CAD build for the part. Positions are in the model's coordinates, mm. A direction names the side the tool comes from. Round coordinates to 2 decimals unless told otherwise and drop trailing zeros. Loops run counter-clockwise (first coordinate to the right, second up) from the corner with the lowest first, then second, coordinate; pieces in that order, holes last.
```python
from build123d import *

# Parameters (mm, degrees)
SKETCH1_W                       = 69.85
SKETCH1_H                       = 25.4
BASE_FLANGE1_DEPTH              = 4.55422
F_7_32_0_21875_DIAMETER_HOLE1_D = 5.55625
BREAK_CORNER1_DEPTH             = 4.55422
SKETCH4_W                       = 34.925
SKETCH4_H                       = 3.175
TAB1_DEPTH                      = 4.55422
FILLET1_R                       = 9.525
CUT_EXTRUDE1_REACH              = 40.633
SKETCH7_R                       = 9.525
CUT_EXTRUDE3_DEPTH              = 2.38125
F_9_32_0_28125_DIAMETER_HOLE1_D = 7.14375
FILLET3_R                       = 12.7
CUT_EXTRUDE4_START              = -2.17297
CUT_EXTRUDE4_DEPTH              = 2.17297


# Read off the part's stored shape, not the designer's step: Break-Corner1
# Sheet-metal steps are written as plain solids
with BuildPart() as part:
    # Sketch1 → Base-Flange1 (new body)
    with BuildSketch(Plane.XY):
        Rectangle(SKETCH1_W, SKETCH1_H)
    extrude(amount=BASE_FLANGE1_DEPTH)

    # 7/32 (0.21875) Diameter Hole1 (through all)
    with Locations(Plane.XY.offset(4.55422)):
        with Locations((-28.575, 6.35), (-28.575, -6.35), (28.575, 6.35), (28.575, -6.35)):
            Hole(F_7_32_0_21875_DIAMETER_HOLE1_D / 2)

    # Break-Corner1 outline → Break-Corner1 (cut)
    with BuildSketch(Plane.XY):
        with BuildLine():
            Line((34.925, -12.7), (34.925, -9.525))
            ThreePointArc((34.925, -9.525), (33.99506403, -11.77006403), (31.75, -12.7))
            Line((31.75, -12.7), (34.925, -12.7))
        make_face()
        with BuildLine():
            ThreePointArc((31.75, 12.7), (33.99506403, 11.77006403), (34.925, 9.525))
            Line((34.925, 9.525), (34.925, 12.7))
            Line((34.925, 12.7), (31.75, 12.7))
        make_face()
        with BuildLine():
            Line((-34.925, -12.7), (-31.75, -12.7))
            ThreePointArc((-31.75, -12.7), (-33.99506403, -11.77006403), (-34.925, -9.525))
            Line((-34.925, -9.525), (-34.925, -12.7))
        make_face()
        with BuildLine():
            ThreePointArc((-34.925, 9.525), (-33.99506403, 11.77006403), (-31.75, 12.7))
            Line((-31.75, 12.7), (-34.925, 12.7))
            Line((-34.925, 12.7), (-34.925, 9.525))
        make_face()
    extrude(amount=BREAK_CORNER1_DEPTH, mode=Mode.SUBTRACT)

    # Sketch4 → Tab1 (add)
    with BuildSketch(Plane(origin=(0, 0, 0), x_dir=(-1, 0, 0), z_dir=(0, 0, -1))):
        with Locations((0, -14.2875)):
            Rectangle(SKETCH4_W, SKETCH4_H)
    extrude(amount=-TAB1_DEPTH)

    # Fillet1
    # the kernel refuses this fillet: 9.525 mm, written as the material it adds along each edge
    with BuildSketch(Plane(origin=(-17.4625, -12.7, 0), x_dir=(-1, 0, 0), z_dir=(0, 0, 1))) as fillet1_piece_1:
        with BuildLine():
            CenterArc((7.099515829, 9.525), FILLET1_R, 221.810314896, 48.189685104)
            Line((0, 3.175), (-0.141990317, 3.048))
            ThreePointArc((-0.141990317, 3.048), (-0.1905, 1.5875), (-0.1905, 0))
            Line((-0.1905, 0), (0, -0.1905))
            Line((0, -0.1905), (7.099515829, -0.1905))
            Line((7.099515829, -0.1905), (7.099515829, 0))
        make_face()
    extrude(amount=4.55422)
    with BuildSketch(Plane(origin=(17.4625, -12.7, 0), x_dir=(1, 0, 0), z_dir=(0, 0, 1))) as fillet1_piece_2:
        with BuildLine():
            CenterArc((7.099515829, -9.525), FILLET1_R, 90, 48.189685104)
            Line((0, -3.175), (-0.141990317, -3.048))
            ThreePointArc((-0.141990317, -3.048), (-0.1905, -1.5875), (-0.1905, 0))
            Line((-0.1905, 0), (0, 0.1905))
            Line((0, 0.1905), (7.099515829, 0.1905))
            Line((7.099515829, 0.1905), (7.099515829, 0))
        make_face()
    extrude(amount=4.55422)

    # Sketch5 → Cut-Extrude1 (cut, up to next)
    with BuildSketch(Plane(origin=(0, 0, 0), x_dir=(-1, 0, 0), z_dir=(0, 0, -1)), mode=Mode.PRIVATE) as cut_extrude1_sk1:
        with BuildLine():
            Line((-8.064231886, 9.525), (8.064231886, 9.525))
            ThreePointArc((8.064231886, 9.525), (9.864287689, 9.69663568), (11.599471303, 10.205357143))
            ThreePointArc((11.599471303, 10.205357143), (17.961811219, 12.070669174), (24.562015829, 12.7))
            Line((24.562015829, 12.7), (-24.562015829, 12.7))
            ThreePointArc((-24.562015829, 12.7), (-17.961811219, 12.070669174), (-11.599471303, 10.205357143))
            ThreePointArc((-11.599471303, 10.205357143), (-9.864287689, 9.69663568), (-8.064231886, 9.525))
        make_face()
    cut_extrude1_tool1 = extrude(cut_extrude1_sk1.sketch, amount=-CUT_EXTRUDE1_REACH, mode=Mode.PRIVATE) & part.part
    add(cut_extrude1_tool1.solids().sort_by_distance((0, 11.328032, 0))[0], mode=Mode.SUBTRACT)

    # Sketch7 → Cut-Extrude3 (cut)
    with BuildSketch(Plane(origin=(0, 0, 0), x_dir=(-1, 0, 0), z_dir=(0, 0, -1))):
        with Locations((0, -3.175)):
            Circle(SKETCH7_R)
    extrude(amount=-CUT_EXTRUDE3_DEPTH, mode=Mode.SUBTRACT)

    # 9/32 (0.28125) Diameter Hole1 (through all)
    with Locations(Plane(origin=(0, 0, 2.38125), x_dir=(-1, 0, 0), z_dir=(0, 0, -1))):
        with Locations((0, -3.175)):
            Hole(F_9_32_0_28125_DIAMETER_HOLE1_D / 2)

    # Fillet3
    fillet3_edges = [part.edges().sort_by_distance(p)[0] for p in [
        (17.4625, -15.875, 2.27711),
        (-17.4625, -15.875, 2.27711),
    ]]
    fillet(fillet3_edges, radius=FILLET3_R)

    # Sketch10 → Cut-Extrude4 (cut)
    with BuildSketch(Plane.XY.offset(4.55422).offset(CUT_EXTRUDE4_START)):
        with BuildLine():
            Line((3.571875, -2.38125), (3.571875, -5.55625))
            ThreePointArc((3.571875, -5.55625), (0, -9.128125), (-3.571875, -5.55625))
            Line((-3.571875, -5.55625), (-3.571875, -2.38125))
            ThreePointArc((-3.571875, -2.38125), (0, 1.190625), (3.571875, -2.38125))
        make_face()
    extrude(amount=CUT_EXTRUDE4_DEPTH, mode=Mode.SUBTRACT)


solid = part.part
```
Item 1: Flat gauge pins, fed straight in: P1, Ø1.4, axis at x = -1, z = 1.5, coming from the +Y side (3 decimals); P2, Ø5.5, axis at x = 3, y = -1, coming from the -Z side; P3, Ø2, axis at x = 26, z = 0.5, coming from the -Y side; P4, Ø4.5, axis at x = 28.575, y = -6.35, coming from the +Z side. Where does each tip first touch, or does it go through?
Answers follow:
P1: stops at y = 9.525
P2: stops at z = 2.38
P3: stops at y = -12.7
P4: passes through
Item 2: 3-axis set-ups, long thin cutter, end or side, ignore diameter. For faces 1 (the cylindrical face through (2.065, -12.473, 1.174)), 2 (the flat face through (28, -12.7, 2)), 3 (the flat face through (-3.572, -4, 3)), 4 (the flat face through (-28, -12.7, 2)): which of +Z, -Z, +X, -X, +Y, -Y reach the whole face in a straight line?
Answers follow:
face 1: -Z
face 2: +Z, -Z, +X, -Y
face 3: +Z, -Z
face 4: +Z, -Z, -X, -Y
Item 3: Cut at D-D, the plane y = -0.5. Give the cut face in (x, z) (3 decimals), plus the area to 3 significant figures.
Answers follow:
outline: (-34.925, 0) - (-9.142, 0) - (-9.142, 2.381) - (-3.036, 2.381) - (-3.036, 4.554) - (-34.925, 4.554) - close; (3.036, 2.381) - (9.142, 2.381) - (9.142, 0) - (34.925, 0) - (34.925, 4.554) - (3.036, 4.554) - close
area: 261 mm2
Item 4: Cut at A-A, the plane x = 0. Give the cut face in (y, z) (3 decimals).
Answers follow:
outline: (-15.875, 0) - (-12.7, 0) - (-12.7, 2.381) - (-9.128, 2.381) - (-9.128, 4.554) - (-15.875, 4.554) - close; (1.191, 2.381) - (6.35, 2.381) - (6.35, 0) - (9.525, 0) - (9.525, 4.554) - (1.191, 4.554) - close
Item 5: Cut at B-B, the plane y = -8.5. Give the cut face in (x, z) (3 decimals).
Answers follow:
outline: (-34.925, 0) - (-30.334, 0) - (-30.334, 4.554) - (-34.925, 4.554) - close; (-26.816, 0) - (-7.897, 0) - (-7.897, 2.381) - (-2.023, 2.381) - (-2.023, 4.554) - (-26.816, 4.554) - close; (2.023, 2.381) - (7.897, 2.381) - (7.897, 0) - (26.816, 0) - (26.816, 4.554) - (2.023, 4.554) - close; (30.334, 0) - (34.925, 0) - (34.925, 4.554) - (30.334, 4.554) - close
Item 6: Probe line 1 (X direction, y = -3.5, z = 1) (3 decimals); line 2 (X direction, y = 4.25, z = 3.5) (3 decimals); line 3 (Y direction, x = -29, z = 1.45). List the from-to ranges inside material, lowest first.
Answers follow:
line 1: x = -34.925 to -9.519, 9.519 to 34.925
line 2: x = -34.925 to -30.394, -26.756 to 26.756, 30.394 to 34.925
line 3: y = -12.7 to -9.1, -3.6 to 3.6, 9.1 to 12.7
Item 7: Two-plate mould, pull along X, no slides. Class faces 5 (the cylindrical face through (-33.97, -11.795, 2.245)), 6 (the flat face through (-4, -3, 2.381)), 7 (the flat face through (8.3, 1.8, 0)), 8 (the cylindrical face through (-0.08, 1.19, 3.45)): released by +X, released by -X, zero draft, split by the parting line, or undercut.
Answers follow:
face 5: released by -X
face 6: undercut
face 7: zero draft
face 8: undercut
Item 8: Cut at C-C, the plane z = 3.35. Give the cut face in (x, y) (3 decimals).
Answers follow:
outline: (-34.925, -9.525) arc R3.175 ccw to (-31.75, -12.7) - (-24.562, -12.7) arc R9.525 cw to (-19.656, -14.061) arc R12.7 ccw to (-13.114, -15.875) - (13.114, -15.875) arc R12.7 ccw to (19.656, -14.061) arc R9.525 cw to (24.562, -12.7) - (31.75, -12.7) arc R3.175 ccw to (34.925, -9.525) - (34.925, 9.525) arc R3.175 ccw to (31.75, 12.7) - (24.562, 12.7) arc R34.925 ccw to (11.599, 10.205) arc R9.525 cw to (8.064, 9.525) - (-8.064, 9.525) arc R9.525 cw to (-11.599, 10.205) arc R34.925 ccw to (-24.562, 12.7) - (-31.75, 12.7) arc R3.175 ccw to (-34.925, 9.525) - close; hole circle Ø5.556 at (-28.575, -6.35); hole circle Ø5.556 at (-28.575, 6.35); hole (-3.572, -5.556) arc R3.572 ccw to (3.572, -5.556) - (3.572, -2.381) arc R3.572 ccw to (-3.572, -2.381) - close; hole circle Ø5.556 at (28.575, -6.35); hole circle Ø5.556 at (28.575, 6.35)
